Geometry: see drawing. Coordinates: mm, zero at the bounding-box minimum. A direction names the side the tool comes from. Round coordinates to 2 decimals unless told otherwise and drop trailing zeros. Loops run counter-clockwise (first coordinate to the right, second up) from the corner with the lowest first, then second, coordinate; pieces in that order, holes last. Notation, with made-up numbers: (-20.75, -35.75) - (-8.75, -35.75) arc R14 cw to (-8.75, -22.75) - close; hole circle Ø9 at (72.25, 18). An arc over 180 degrees is marked (long way). Use CSV: the item, a comma, the result in double quotes.
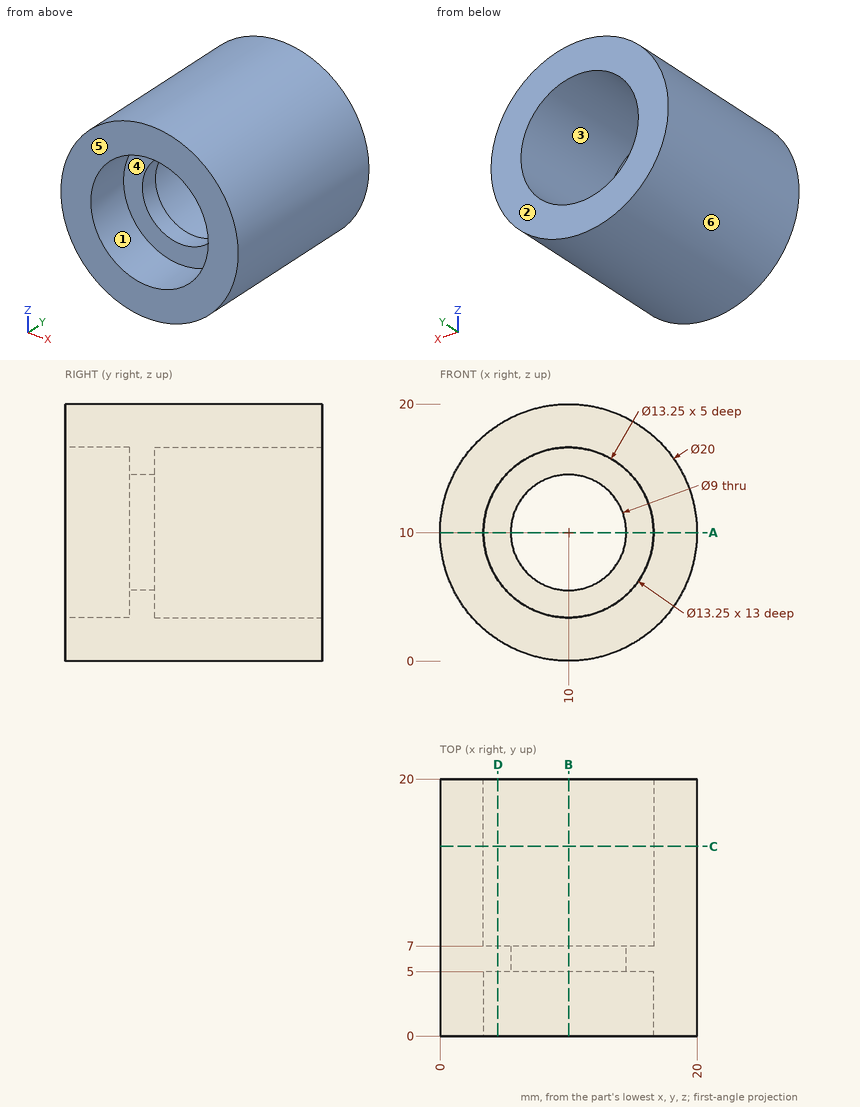
Item 1: Reachability of the marked faces 1, 2 and 3 from +Z, -Z, +X, -X, +Y, -Y: full face, straight path, thin tool, end or side. Return the list, or none.
Final values:
face 1,"-Y"
face 2,"+Z, -Z, +X, -X, +Y"
face 3,"+Y"
Item 2: Section B-B on x = 10. Return the cut outline in (y, z) (3 decimals), plus the area to 4 significant figures.
Final values:
outline,"(0, 0) - (20, 0) - (20, 3.375) - (7, 3.375) - (7, 5.5) - (5, 5.5) - (5, 3.375) - (0, 3.375) - close; (0, 16.625) - (5, 16.625) - (5, 14.5) - (7, 14.5) - (7, 16.625) - (20, 16.625) - (20, 20) - (0, 20) - close"
area,"143.5 mm²"
Item 3: Section A-A on z = 10. Return the cut outline in (x, y) (3 decimals), plus the area to 4 significant figures.
Final values:
outline,"(0, 0) - (3.375, 0) - (3.375, 5) - (5.5, 5) - (5.5, 7) - (3.375, 7) - (3.375, 20) - (0, 20) - close; (14.5, 5) - (16.625, 5) - (16.625, 0) - (20, 0) - (20, 20) - (16.625, 20) - (16.625, 7) - (14.5, 7) - close"
area,"143.5 mm²"
Item 4: Section D-D on x = 4.5. Return the cut outline in (y, z), plus the area to 3 significant figures.
Final values:
outline,"(0, 1.65) - (20, 1.65) - (20, 6.31) - (7, 6.31) - (7, 13.69) - (20, 13.69) - (20, 18.35) - (0, 18.35) - (0, 13.69) - (5, 13.69) - (5, 6.31) - (0, 6.31) - close"
area,"201 mm²"
Item 5: Material intervals for line 1 (Z direction, x = 10, y = 10.5) (3 decimals); line 2 (Z direction, x = 10, y = 5.85); line 3 (Y direction, x = 12, z = 15.75), sorted ascending.
Final values:
line 1,"z = 0 to 3.375, 16.625 to 20"
line 2,"z = 0 to 5.5, 14.5 to 20"
line 3,"y = 5 to 7"
Item 6: Mould query, pull axis Z, two halves, no side actions, for the marked faces 4, 5 and 6. Classes: released by +Z, released by -Z, zero draft, split by the parting line, or undercut.
Final values:
face 4,"undercut"
face 5,"zero draft"
face 6,"split by the parting line"
Item 7: Section C-C on y = 14.75. Return the cut outline in (x, z) (3 decimals), plus the area to 3 significant figures.
Final values:
outline,"circle Ø20 at (10, 10); hole circle Ø13.25 at (10, 10)"
area,"176 mm²"
Item 8: Pin query (flat end, axial travel): P1, Ø10.5, axis at x = 10, z = 10, coming from the +Y side; P2, Ø4, axis at y = 12, z = 14, coming from the +X side; P3, Ø8, axis at x = 3.5, y = 2, coming from the +Z side. Return the tip coordinate at first contact, or that it passes through.
Final values:
P1,"stops at y = 7"
P2,"stops at x = 19.8"
P3,"stops at z = 19.68"
